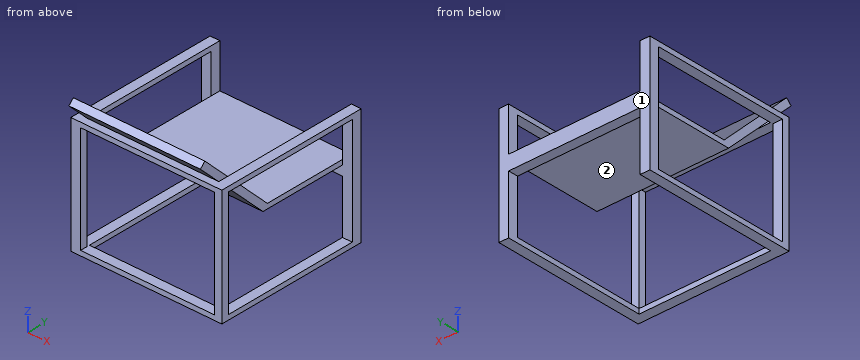
```python
from build123d import *

# Parameters (mm, degrees)
F0_W      = 787.4
F0_H      = 50.8
F1_DEPTH  = 609.6
F2_W      = 711.2
F2_H      = 558.8
F3_DEPTH  = 50.8
F4_W      = 38.1
F4_H      = 609.6
F5_DEPTH  = 736.6
F6_W      = 711.2
F6_H      = 558.8
F7_DEPTH  = 50.8
F8_DEPTH  = 12.7
F10_DEPTH = 736.6
F11_DEPTH = 12.7
F12_W     = 711.2
F12_H     = 558.8
F13_DEPTH = 50.8
F14_W     = 38.1
F14_H     = 50.8
F15_DEPTH = 711.2
F16_DEPTH = 12.7
F17_W     = 685.8
F17_H     = 508
F18_DEPTH = 25.4
F19_SIZE  = 25.39999
F20_W     = 685.8
F20_H     = 35.9210244843
F21_DEPTH = 508


# Not quite as in the source:
# - a fillet or chamfer is up to 0.001 mm smaller than in the source, because OpenCascade refuses the exact size


with BuildPart() as f1:
    # F0 (on Top) → F1 (new body)
    with BuildSketch(Plane.XY):
        with Locations((273.7565302372, -36.9653456569)):
            Rectangle(F0_W, F0_H)
    extrude(amount=F1_DEPTH)

    # F2 (on face) → F3 (cut)
    with BuildSketch(Plane.XZ.offset(62.3653456569)):
        with Locations((273.7565302372, 304.8)):
            Rectangle(F2_W, F2_H)
    extrude(amount=-F3_DEPTH, mode=Mode.SUBTRACT)

    # F4 (on face) → F5 (join)
    with BuildSketch(Plane(origin=(0, -11.5653456569, 0), x_dir=(-1, 0, 0), z_dir=(0, 1, 0))):
        with Locations((-648.4065302372, 304.8)):
            Rectangle(F4_W, F4_H)
    extrude(amount=F5_DEPTH)

    # F6 (on face) → F7 (cut)
    with BuildSketch(Plane.YZ.offset(667.4565302372)):
        with Locations((331.3346543431, 304.8)):
            Rectangle(F6_W, F6_H)
    extrude(amount=-F7_DEPTH, mode=Mode.SUBTRACT)

    # F8 (add): a face of the model
    f8_faces = [f1.faces().sort_by_distance(p)[0] for p in [
        (629.3565302372, -2.0040083027, 12.7),
    ]]
    extrude(f8_faces, amount=F8_DEPTH)

    # F9 (on face) → F10 (join)
    with BuildSketch(Plane(origin=(0, -11.5653456569, 0), x_dir=(-1, 0, 0), z_dir=(0, 1, 0))):
        Polygon((119.9434697628, 0), (119.9434697628, 609.6), (81.8434697628, 609.6), (81.8434697628, 584.2), (81.8434697628, 25.4), (81.8434697628, 0), align=None)
    extrude(amount=F10_DEPTH)

    # F11 (add): a face of the model
    f11_faces = [f1.faces().sort_by_distance(p)[0] for p in [
        (-81.8434697628, 333.3254651539, 304.8),
    ]]
    extrude(f11_faces, amount=F11_DEPTH)

    # F12 (on face) → F13 (cut)
    with BuildSketch(Plane(origin=(-119.9434697628, 0, 0), x_dir=(0, -1, 0), z_dir=(-1, 0, 0))):
        with Locations((-331.3346543431, 304.8)):
            Rectangle(F12_W, F12_H)
    extrude(amount=-F13_DEPTH, mode=Mode.SUBTRACT)

    # F14 (on face) → F15 (join)
    with BuildSketch(Plane.YZ.offset(-69.1434697628)):
        with Locations((705.9846543431, 330.2)):
            Rectangle(F14_W, F14_H)
    extrude(amount=F15_DEPTH)

    # F16 (add): a face of the model
    f16_faces = [f1.faces().sort_by_distance(p)[0] for p in [
        (273.7565302372, 725.0346543431, 313.944),
    ]]
    extrude(f16_faces, amount=F16_DEPTH)

    # F17 (on face) → F18 (join)
    with BuildSketch(Plane.XY.offset(355.6)):
        with Locations((273.7565302372, 483.7346543431)):
            Rectangle(F17_W, F17_H)
    extrude(amount=F18_DEPTH)

    # F19 (size 25.4 in the source; OpenCascade refuses exactly that, so slightly less here)
    f19_edges = [f1.edges().sort_by_distance(p)[0] for p in [
        (273.75653, 229.734654, 381),
    ]]
    chamfer(f19_edges, length=F19_SIZE)

    # F20 (on face) → F21 (join)
    with BuildSketch(Plane(origin=(0, -62.9326728284, 62.9326728284), x_dir=(1, 0, 0), z_dir=(0, -0.7071067812, 0.7071067812))):
        with Locations((273.7565302372, 431.8546155916)):
            Rectangle(F20_W, F20_H)
    extrude(amount=F21_DEPTH)


solid = f1.part
```
For this review, take the finished solid that the model builds, in its own axes (mm). Face numbers are marked on the shaded views. A direction names the side the tool comes from. Coordinates: 2 decimals unless noted, no trailing zeros. Loops run counter-clockwise (first coordinate to the right, second up) from the corner with the lowest first, then second, coordinate; pieces in that order, holes last. Notation, with made-up numbers: (40, 45) - (80, 45) arc R17 cw to (80, 52) - close; hole circle Ø7 at (-36, 64.5). An arc over 180 degrees is marked (long way). Use one line per item in the form item = value. Start each with the question number.
1) Take a section at A-A (y = 448). State the section outline as (x, z) points, plus the area to 3 significant figures.
2) To check wall thickness, follow probe 1 along X at (y, z) = (699.5, 498.5); probe 2 along Z at (x, y) = (51, 315); probe 3 along X at (y, z) = (413, 370.5). State the ranges of each line that lie inside material, in increasing order. Write a range as from..to.
3) For pin 1 (6 mm diameter, centred on x = 110.5, z = 631.5, fed in from -Y); pin 2 (1.5 mm diameter, centred on x = 245, y = 67.5, fed in from -Z); pin 3 (14 mm diameter, centred on x = 192, z = 589, fed in from +Y), all flat-tipped, find the tip position at first contact; note any pin that passes through.
4) For the marked faces 1 and 2, list the 3-axis set-ups (+Z, -Z, +X, -X, +Y, -Y) from which the entire face can be reached by the end or side of a thin tool; tool diameter is ignored.
5) Take a section at D-D (z = 477.5). State the section outline as (x, y) points.
6) Take a section at C-C (z = 140). State the section outline as (x, y) points.
7) Take a section at B-B (x = 525). State the section outline as (y, z) points.
From the geometry:
q1.outline = (-119.94, 0) - (-69.14, 0) - (-69.14, 25.4) - (-119.94, 25.4) - close; (-119.94, 584.2) - (-69.14, 584.2) - (-69.14, 609.6) - (-119.94, 609.6) - close; (-69.14, 355.6) - (616.66, 355.6) - (616.66, 381) - (-69.14, 381) - close; (616.66, 0) - (667.46, 0) - (667.46, 25.4) - (616.66, 25.4) - close; (616.66, 584.2) - (667.46, 584.2) - (667.46, 609.6) - (616.66, 609.6) - close
q1.area = 22,600 mm2
q2.probe_1 = -119.94..-69.14, 616.66..667.46
q2.probe_2 = 355.6..381
q2.probe_3 = -69.14..616.66
q3.pin_1 = -49.17
q3.pin_2 = 517.08
q3.pin_3 = 54.13
q4.face_1 = +Z, -Z, +X, -X, +Y
q4.face_2 = -Z, +X, -X, -Y
q5.outline = (-119.94, -62.37) - (-69.14, -62.37) - (-69.14, -24.27) - (-119.94, -24.27) - close; (-119.94, 686.93) - (-69.14, 686.93) - (-69.14, 737.73) - (-119.94, 737.73) - close; (-69.14, 107.83) - (616.66, 107.83) - (616.66, 158.63) - (-69.14, 158.63) - close; (616.66, 686.93) - (667.46, 686.93) - (667.46, 737.73) - (616.66, 737.73) - close; (629.36, -62.37) - (667.46, -62.37) - (667.46, -24.27) - (629.36, -24.27) - close
q6.outline = (-119.94, -62.37) - (-69.14, -62.37) - (-69.14, -24.27) - (-119.94, -24.27) - close; (-119.94, 686.93) - (-69.14, 686.93) - (-69.14, 737.73) - (-119.94, 737.73) - close; (616.66, 686.93) - (667.46, 686.93) - (667.46, 737.73) - (616.66, 737.73) - close; (629.36, -62.37) - (667.46, -62.37) - (667.46, -24.27) - (629.36, -24.27) - close
q7.outline = (-129.48, 714.81) - (-24.27, 609.6) - (-62.37, 609.6) - (-62.37, 584.2) - (-11.57, 584.2) - (-11.57, 596.9) - (229.73, 355.6) - (686.93, 355.6) - (686.93, 304.8) - (737.73, 304.8) - (737.73, 381) - (255.13, 381) - (-104.08, 740.21) - close; (-62.37, 0) - (-11.57, 0) - (-11.57, 25.4) - (-62.37, 25.4) - close
